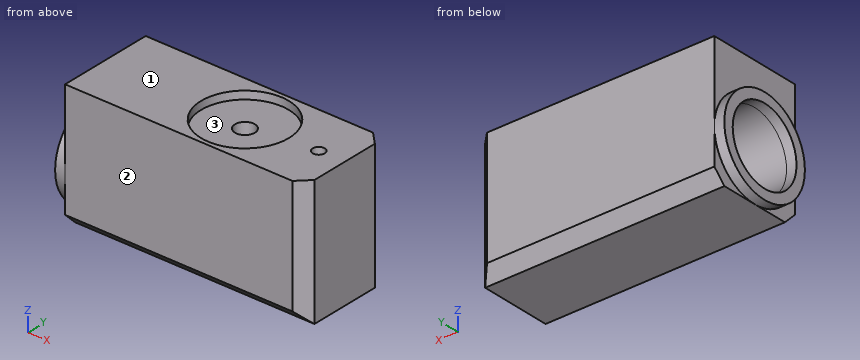
```python
from build123d import *

# Parameters (mm, degrees)
SKETCH1_W             = 60
SKETCH1_H             = 24
BOSS_EXTRUDE1_DEPTH   = 16
CHAMFER1_SIZE         = 3
SKETCH2_R             = 11
CUT_EXTRUDE1_DEPTH    = 2
SKETCH3_R             = 12
SKETCH3_R_2           = 9.5
BOSS_EXTRUDE2_DEPTH   = 2.5
CUT_EXTRUDE2_START    = -53
SKETCH4_R             = 9.5
CUT_EXTRUDE2_DEPTH    = 53
CHAMFER2_SIZE         = 3
SKETCH5_R             = 1.5
CUT_EXTRUDE3_DEPTH    = 12
M6_TAPPED_HOLE1_D     = 5
M6_TAPPED_HOLE1_DEPTH = 12
M6_TAPPED_HOLE1_TIP   = 1.502151548


with BuildPart() as part:
    # Sketch1 → Boss-Extrude1 (new, symmetric)
    with BuildSketch(Plane.XY):
        Rectangle(SKETCH1_W, SKETCH1_H)
    extrude(amount=BOSS_EXTRUDE1_DEPTH, both=True)

    # Chamfer1
    chamfer1_edges = [part.edges().sort_by_distance(p)[0] for p in [
        (30, -12, 0),
        (30, 12, 0),
    ]]
    chamfer(chamfer1_edges, length=CHAMFER1_SIZE)

    # Sketch2 → Cut-Extrude1 (cut)
    with BuildSketch(Plane.XY.offset(16)):
        with Locations((5, 0)):
            Circle(SKETCH2_R)
    extrude(amount=-CUT_EXTRUDE1_DEPTH, mode=Mode.SUBTRACT)

    # Sketch3 → Boss-Extrude2 (add, symmetric)
    with BuildSketch(Plane.ZY.offset(30)):
        with Locations(Location((-4, 0, 0), (0, 0, 270))):
            Circle(SKETCH3_R)
        with Locations(Location((-4, 0, 0), (0, 0, 90))):
            Circle(SKETCH3_R_2, mode=Mode.SUBTRACT)
    extrude(amount=BOSS_EXTRUDE2_DEPTH, both=True)

    # Sketch4 → Cut-Extrude2 (cut)
    with BuildSketch(Plane.ZY.offset(30).offset(CUT_EXTRUDE2_START)):
        with Locations(Location((-4, 0, 0), (0, 0, 270))):
            Circle(SKETCH4_R)
    extrude(amount=CUT_EXTRUDE2_DEPTH, mode=Mode.SUBTRACT)

    # Chamfer2
    chamfer2_edges = [part.edges().sort_by_distance(p)[0] for p in [
        (-1.5, -12, -16),
        (-1.5, 12, -16),
    ]]
    chamfer(chamfer2_edges, length=CHAMFER2_SIZE)

    # Sketch5 → Cut-Extrude3 (cut)
    with BuildSketch(Plane.XY.offset(16)):
        with Locations((23.5, 0)):
            Circle(SKETCH5_R)
    extrude(amount=-CUT_EXTRUDE3_DEPTH, mode=Mode.SUBTRACT)

    # M6 Tapped Hole1
    with Locations(Plane.XY.offset(14)):
        with Locations((5, 0)):
            Hole(M6_TAPPED_HOLE1_D / 2, depth=M6_TAPPED_HOLE1_DEPTH)
            with Locations((0, 0, -(M6_TAPPED_HOLE1_DEPTH + M6_TAPPED_HOLE1_TIP / 2))):  # 118° drill point
                Cone(0, M6_TAPPED_HOLE1_D / 2, M6_TAPPED_HOLE1_TIP, mode=Mode.SUBTRACT)


solid = part.part
```
Model file for the job. Use its own axes, mm. Face numbers are marked on the shaded views. Give positions to 0.01 mm unless a question says otherwise; leave off trailing zeros. Loops run counter-clockwise (first coordinate to the right, second up) from the corner with the lowest first, then second, coordinate; pieces in that order, holes last. Notation, with made-up numbers: (-36.75, -9) -> (20.25, -9) arc R11 ccw to (20.25, 2) -> close; hole circle Ø7 at (7.25, 52.25). An arc over 180 degrees is marked (long way). Use CSV: the item, a comma, the result in double quotes. Start each with the question number.
1) Wall check: line 1 (X direction, y = 0, z = 8.5); line 2 (Z direction, x = -23, y = 7.75); line 3 (Y direction, x = -16, z = -4). Give the ranges that are in metal, low to high.
2) Slice it at C-C on x = 5. Give the cut face in (y, z), plus the area to 3 significant figures.
3) Mould opens along Y. For the marked faces 1, 2 and 3 say: released by +Y, released by -Y, zero draft, split by the parting line, or undercut.
4) Slice it at B-B on z = 13. Give the cut face in (x, y).
5) Slice it at D-D on z = 7. Give the cut face in (x, y), plus the area to 3 significant figures.
6) Slice it at A-A on x = 21. Give the cut face in (y, z).
7) Flat gauge pins, fed straight in: pin 1 Ø3.5 at (y, z) = (7.5, -9.5) entering from -X; pin 2 Ø1.5 at (y, z) = (-3.5, -1) entering from -X; pin 3 Ø1 at (y, z) = (8, 7.5) entering from -X; pin 4 Ø6.5 at (x, y) = (6, -1) entering from +Z. Where does each tip first touch, or does it go through?
Computed values:
1,line 1,"x = -30 to 2.5, 7.5 to 22, 25 to 30"
1,line 2,"z = -16 to -9.49, 1.49 to 16"
1,line 3,"y = -12 to -9.5, 9.5 to 12"
2,outline,"(-12, -13) -> (-9, -16) -> (9, -16) -> (12, -13) -> (12, 16) -> (11, 16) -> (11, 14) -> (2.5, 14) -> (2.5, 5.17) arc R9.5 cw (long way) to (-2.5, 5.17) -> (-2.5, 14) -> (-11, 14) -> (-11, 16) -> (-12, 16) -> close"
2,area,"388 mm^2"
3,face 1,"zero draft"
3,face 2,"released by -Y"
3,face 3,"undercut"
4,outline,"(-30, -12) -> (27, -12) -> (30, -9) -> (30, 9) -> (27, 12) -> (-30, 12) -> close; hole circle Ø5 at (5, 0); hole circle Ø3 at (23.5, 0)"
5,outline,"(-32.5, -4.8) -> (-30, -4.8) -> (-30, -12) -> (27, -12) -> (30, -9) -> (30, 9) -> (27, 12) -> (-30, 12) -> (-30, 4.8) -> (-32.5, 4.8) -> close; hole circle Ø5 at (5, 0); hole circle Ø3 at (23.5, 0)"
5,area,"1,430 mm^2"
6,outline,"(-12, -13) -> (-9, -16) -> (9, -16) -> (12, -13) -> (12, 16) -> (-12, 16) -> close; hole circle Ø19 at (0, -4)"
7,pin 1,"stops at x = -32.5"
7,pin 2,"stops at x = 23"
7,pin 3,"stops at x = -30"
7,pin 4,"stops at z = 14"
